Autodesk Inventor part; units mm, degrees
ref_plane "YZ Plane" through (0, 0, 0) normal (1, 0, 0) x (0, 1, 0)
ref_plane "XZ Plane" through (0, 0, 0) normal (0, 1, 0) x (-1, 0, 0)
ref_plane "XY Plane" through (0, 0, 0) normal (0, 0, 1) x (1, 0, 0)
ref_plane "작업 평면1" through (0, 0, 0) normal (0, 0, 1) x (1, 0, 0)
sketch "스케치1" plane through (0, 0, 0) normal (0, 0, 1) x (1, 0, 0)
  line L0 (-35, -17.5) -> (35, -17.5)
  line L1 (35, -17.5) -> (35, 17.5)
  line L2 (35, 17.5) -> (-35, 17.5)
  line L3 (-35, 17.5) -> (-35, -17.5)
  line L4 (35, -17.5) -> (-35, -17.5)
  line L5 (-35, -17.5) -> (-35, -23.5)
  line L6 (35, -23.5) -> (-35, -23.5)
  line L7 (35, -17.5) -> (35, -23.5)
  line L8 (35, 0) -> (10, 0)
  line L9 (-35, 0) -> (-10, 0)
  line L10 (10, 0) -> (-10, 0)
  line L11 (10, 0) -> (10, 17.5)
  line L12 (-10, 0) -> (-10, 17.5)
  line L13 (10, 17.5) -> (-10, 17.5)
  line L14 (-10, 17.5) -> (-10, 7.5)
  line L15 (-10, 7.5) -> (10, 7.5)
  line L16 (10, 7.5) -> (10, 17.5)
  point P0 (0, 0)
  dimension "d0" = 25
  dimension "d1" = 25
  dimension "d2" = 20
  dimension "d3" = 10
extrude "돌출1" add sketch "스케치1" along normal blind 3 contours L2 L11 L15 L12
sketch "스케치2" plane through (0, 0, 3) normal (0, 0, 1) x (1, 0, 0)
  line L0 (10, 7.5) -> (10, 17.5)
  line L1 (10, 17.5) -> (-10, 17.5)
  line L2 (-10, 17.5) -> (-10, 7.5)
  line L3 (-10, 7.5) -> (10, 7.5)
  line L4 (10, 17.5) -> (-10, 17.5)
  line L5 (-10, 17.5) -> (-10, 14.5)
  line L6 (-10, 14.5) -> (10, 14.5)
  line L7 (10, 14.5) -> (10, 17.5)
  point P0 (0, 0)
  point P1 (10, 14.5)
  dimension "d6" = 3
extrude "돌출2" add sketch "스케치2" along normal blind 10 contours L6 L2 L1 L0
sketch "스케치3" plane through (0, 0, 3) normal (0, 0, 1) x (1, 0, 0)
  line L0 (10, 14.5) -> (-10, 14.5)
  line L1 (-10, 14.5) -> (-10, 7.5)
  line L2 (-10, 7.5) -> (10, 7.5)
  line L3 (10, 7.5) -> (10, 14.5)
  line L4 (10, 11) -> (4, 11)
  line L5 (-10, 11) -> (-4, 11)
  circle A0 centre (4, 11) radius 1.25
  circle A1 centre (-4, 11) radius 1.25
  point P0 (0, 0)
  dimension "d9" = 6
  dimension "d10" = 6
  dimension "d11" = 2.5
  dimension "d12" = 2.5
extrude "돌출3" cut sketch "스케치3" against normal blind 10 contours A1 | A0
sketch "스케치4" plane through (-10, 14.5, 3) normal (0, -1, 0) x (1, 0, 0)
  line L0 (20, 0) -> (0, 0)
  line L1 (20, 0) -> (20, 10)
  line L2 (0, 10) -> (20, 10)
  line L3 (0, 0) -> (0, 10)
  line L4 (20, 5) -> (14, 5)
  line L5 (0, 5) -> (6, 5)
  circle A0 centre (14, 5) radius 1.25
  circle A1 centre (6, 5) radius 1.25
  point P0 (10, -3)
  dimension "d15" = 6
  dimension "d16" = 6
  dimension "d17" = 2.5
  dimension "d18" = 2.5
extrude "돌출4" cut sketch "스케치4" against normal blind 10 contours A0 | A1
properties part number "63" material "LCP 플라스틱"
Model file for the job. Use its own axes, mm. A direction names the side the tool comes from. Coordinates: 2 decimals unless noted, no trailing zeros. Write each loop counter-clockwise with the first axis right and the second up, starting at its lowest first coordinate (ties: lowest second). Pieces come first, ordered by that corner, then holes. Notation, with made-up numbers: (62, 81) - (108, 81) arc R13 ccw to (108, 93) - close; hole circle Ø11 at (64.25, -24). An arc over 180 degrees is marked (long way). Write each question's results on one line, items separated by ' | '. Start each with the question number.
1) Mould opens along Z. For faces 3 (the face through (0, 11, 3)), 4 (the face through (-4.27, 15.98, 6.78)), 5 (the face through (4.672, 12.054, 1.521)) say: pulls with the +Z half, pulls with the -Z half, needs draft (parallel to the pull), parting line crosses it, or undercut.
2) Probe line 1 along Y through (x, z) = (-4, 1); line 2 along Z through (x, y) = (4, 15.3); line 3 along Y through (x, z) = (-7.5, 5). List the from-to ranges inside material, lowest first. Write a range as from..to.
3) Cut at B-B (x = 4). Write the cut outline in (y, z), then the cut area to 3 significant figures.
4) Flat gauge pins, fed straight in: P1, Ø3, axis at x = 4, z = 8, coming from the -Y side; P2, Ø1, axis at x = -2.5, y = 13, coming from the +Z side. Where does each tip first touch, or does it go through?
5) Cut at D-D (x = -2.5). Write the cut outline in (y, z).
6) 3-axis set-ups, long thin cutter, end or side, ignore diameter. For faces 1 (the face through (0, 14.5, 8)), 2 (the face through (0, 13, 0)): which of +Z, -Z, +X, -X, +Y, -Y reach the whole face in a straight line?
7) Cut at A-A (z = 8). Write the cut outline in (x, y), then the cut area to 3 significant figures.
8) Cut at C-C (y = 11). Write the cut outline in (x, z).
Returned:
1) face 3: pulls with the +Z half | face 4: undercut | face 5: needs draft
2) line 1: 7.5..9.75, 12.25..17.5 | line 2: 0..6.75, 9.25..13 | line 3: 14.5..17.5
3) outline: (7.5, 0) - (9.75, 0) - (9.75, 3) - (7.5, 3) - close; (12.25, 0) - (17.5, 0) - (17.5, 6.75) - (14.5, 6.75) - (14.5, 3) - (12.25, 3) - close; (14.5, 9.25) - (17.5, 9.25) - (17.5, 13) - (14.5, 13) - close | area: 45.0 mm^2
4) P1: y = 14.5 | P2: z = 3
5) outline: (7.5, 0) - (17.5, 0) - (17.5, 13) - (14.5, 13) - (14.5, 3) - (7.5, 3) - close
6) face 1: +Z, +X, -X, -Y | face 2: -Z, +X, -X, +Y, -Y
7) outline: (-10, 14.5) - (-5.25, 14.5) - (-5.25, 17.5) - (-10, 17.5) - close; (-2.75, 14.5) - (2.75, 14.5) - (2.75, 17.5) - (-2.75, 17.5) - close; (5.25, 14.5) - (10, 14.5) - (10, 17.5) - (5.25, 17.5) - close | area: 45.0 mm^2
8) outline: (-10, 0) - (-5.25, 0) - (-5.25, 3) - (-10, 3) - close; (-2.75, 0) - (2.75, 0) - (2.75, 3) - (-2.75, 3) - close; (5.25, 0) - (10, 0) - (10, 3) - (5.25, 3) - close
